from build123d import *

# Parameters (mm, degrees)
SKETCH3_R           = 3.174999999999997
BOSS_EXTRUDE2_DEPTH = 30
SKETCH3_6_R         = 6.249999999999999
SKETCH3_6_R_2       = 3.174999999999996
BOSS_EXTRUDE3_DEPTH = 15
FILLET1_R           = 10
CHAMFER1_SIZE       = 1


with BuildPart() as part:
    # Sketch3 → Boss-Extrude2 (new body)
    with BuildSketch(Plane(origin=(0, 0, 0), x_dir=(1, 0, 0), z_dir=(0, 1, 0))):
        with BuildLine():
            ThreePointArc((-9.29e-15, 31), (-4.229978997044333, 32.64893733094583), (-6.227967505338837, 36.72567114093955))
            ThreePointArc((-6.227967505338856, 36.72567114093959), (-28.456583505173906, 24.03716612275798), (-37.249999999999986, -3.82e-15))
            Line((-37.25, 0), (-41.75, -5.5e-16))
            Line((-41.75, -5.5e-16), (-41.75, -3.000000000000001))
            Line((-41.75, -3.000000000000001), (-40.25, -3.000000000000001))
            Line((-40.25, -3.000000000000001), (-40.25, -1.5000000000000004))
            Line((-40.25, -1.5000000000000004), (-37.21978640454563, -1.5000000000000004))
            ThreePointArc((-37.21978640454562, -1.5000000000000002), (-36.52259085251633, -7.325493663889764), (-34.919347931756114, -12.969257496902395))
            ThreePointArc((-34.91934793175618, -12.969257496902411), (-37.67210506462307, -21.75000000000005), (-28.691380426417297, -23.75641364403726))
            ThreePointArc((-28.691380426417272, -23.756413644037238), (-16.975861979154317, -33.15693909372066), (-2.5, -37.166012699777184))
            Line((-2.4999999999999982, -37.1660126997772), (-2.4999999999999982, -44.1660126997772))
            Line((-2.4999999999999982, -44.1660126997772), (-3.9999999999999982, -44.1660126997772))
            Line((-3.9999999999999982, -44.1660126997772), (-3.9999999999999982, -45.6660126997772))
            Line((-3.9999999999999982, -45.6660126997772), (1.8e-15, -45.6660126997772))
            Line((1.8e-15, -45.6660126997772), (8.2e-16, -30.99999999999999))
            ThreePointArc((8.2e-16, -30.999999999999986), (-30.999999999999986, -3.39e-15), (-1.128e-14, 30.999999999999993))
        make_face()
        with Locations(Location((-32.25944629097033, -18.62500000000002, 0), (0, 0, 270))):
            Circle(SKETCH3_R, mode=Mode.SUBTRACT)
    extrude(amount=BOSS_EXTRUDE2_DEPTH)

    # Sketch3<6> → Boss-Extrude3 (add)
    with BuildSketch(Plane(origin=(0, 0, 0), x_dir=(1, 0, 0), z_dir=(0, 1, 0))):
        with Locations((-8.14e-15, 37.25)):
            Circle(SKETCH3_6_R)
        with Locations(Location((-8.14e-15, 37.25, 0), (0, 0, 270))):
            Circle(SKETCH3_6_R_2, mode=Mode.SUBTRACT)
    extrude(amount=BOSS_EXTRUDE3_DEPTH)

    # Fillet1
    # the kernel refuses this fillet: 10 mm, written as the material it adds along each edge
    with BuildSketch(Plane(origin=(-28.691380426417282, 0, 23.75641364403725), x_dir=(-0.9506898736636257, 0, 0.3101431348803961), z_dir=(0, 1, 0))) as fillet1_piece_1:
        with BuildLine():
            CenterArc((6.482344939436471, 9.575990594652419), FILLET1_R, 209.4937649075162, 43.761742692679945)
            ThreePointArc((-2.221747837989829, 4.652702169021102), (-1.030276989978153, 2.3648375481367587), (0, 0))
            ThreePointArc((0, 0), (1.8006513720656931, 0.26500587834223527), (3.6013027441313774, -6e-17))
        make_face()
    extrude(amount=30)
    with BuildSketch(Plane(origin=(-34.91934793175615, 0, 12.969257496902403), x_dir=(-0.7439367704475782, 0, 0.6682500142731217), z_dir=(0, 1, 0))) as fillet1_piece_2:
        with BuildLine():
            CenterArc((6.482344939436458, -9.575990594652419), FILLET1_R, 106.74449239980393, 43.76174269267989)
            ThreePointArc((-2.2217478379898448, -4.652702169021106), (-1.0302769899781694, -2.364837548136756), (0, 0))
            ThreePointArc((0, 0), (1.8006513720656803, -0.26500587834223843), (3.601302744131356, 6e-17))
        make_face()
    extrude(amount=30)
    with BuildSketch(Plane(origin=(-6.227967505338847, 0, -36.725671140939575), x_dir=(-0.9719890656078827, 0, 0.23502607586971094), z_dir=(0, 1, 0))) as fillet1_piece_3:
        with BuildLine():
            CenterArc((5.848021683595468, -9.976022963631705), FILLET1_R, 93.96846171792617, 43.7617426926798)
            ThreePointArc((-1.5518361342237537, -3.2497978502371354), (-0.5367780683599742, -1.7390925175521244), (0, 0))
            ThreePointArc((0, 0), (2.5779740557861452, -0.08931446047189494), (5.1559481115722905, 1e-17))
        make_face()
    extrude(amount=15)
    with BuildSketch(Plane(origin=(-37.24999999999999, 0, 1.78e-15), x_dir=(-1, 0, -7.737e-14), z_dir=(0, 1, 0))) as fillet1_piece_4:
        with BuildLine():
            CenterArc((9.164670658683216, -8.845385669716253), FILLET1_R, 117.80520941997419, 51.405137085838774)
            ThreePointArc((-0.6585400627312272, -6.973346374538821), (-0.16500045393500687, -3.5021862698004864), (0, 0))
            Line((0, 0), (4.500000000000192, 0))
        make_face()
    extrude(amount=30)

    # Chamfer1
    chamfer1_edges = [part.edges().sort_by_distance(p)[0] for p in [
        (-7.903771868670522, 0, -37.32519260636591),
        (-38.375294648334496, 0, -2.898249101229199),
        (-38.375294648334496, 30, -2.898249101229199),
        (-36.27645093259372, 0, 11.817729079196308),
        (-36.27645093259372, 30, 11.817729079196308),
        (-30.999999999999986, 0, 5.16e-15),
        (1.31e-15, 0, 38.33300634988859),
        (-2.4999999999999982, 0, 40.6660126997772),
        (-14.640454765554196, 0, 34.25229312407797),
        (-14.640454765554196, 30, 34.25229312407797),
        (-2.4999999999999982, 30, 40.6660126997772),
        (1.31e-15, 30, 38.33300634988859),
        (-30.999999999999986, 30, 5.16e-15),
        (-4.2299789970443324, 30, -32.64893733094583),
        (5.376209478406283, 0, -40.43729848685283),
        (-37.672105064623324, 0, 21.749999999999595),
        (-37.672105064623324, 30, 21.749999999999595),
        (-27.849428165120642, 0, -24.7380648167108),
        (-26.07059740166155, 30, -26.60613559163521),
        (-36.941998560282954, 0, 4.780297310006034),
        (-36.941998560282954, 30, 4.780297310006034),
        (-28.372679063924544, 0, 25.507463527167676),
        (-28.372679063924544, 30, 25.507463527167676),
    ]]
    chamfer(chamfer1_edges, length=CHAMFER1_SIZE)


solid = part.part
Build history of the part. All positions in model axes, mm. A direction names the side the tool comes from. Coordinates: 2 decimals unless noted, no trailing zeros. Order: outer loops, then holes, each group sorted by start corner. A loop starts at its lowest first (then second) coordinate and runs counter-clockwise, first axis right, second up. Notation, with made-up numbers: (76.5, -22) - (112.5, -22) arc R25 cw to (112.5, 17) - close; hole circle Ø1 at (27.25, 44). An arc over 180 degrees is marked (long way). Write each question's results on one line, items separated by ' | '. Start each with the question number.
Item 1: Flat gauge pins, fed straight in: pin 1 (2 mm diameter, centred on x = -18, y = 6, fed in from +Z); pin 2 (2 mm diameter, centred on x = -37.5, y = 13, fed in from +Z); pin 3 (1.7 mm diameter, centred on y = 8, z = 2.5, fed in from +X). Where does each tip first touch, or does it go through?
Item 2: Band-saw the part on A-A on y = 10.5. State how many separate pieces and enclosed holes the cut face has, and give its area (3 significant figures).
Item 3: Wall check: probe 1 along Z at (x, y) = (-3, 27); probe 2 along Z at (x, y) = (-2, 5.5); probe 3 along Z at (x, y) = (-37.5, 26). Give the ranges that are in metal, low to high. Write a range as [from, to].
Item 4: Tool access for faces 4 (the face through (-36.95, 14.8, 4.73)), 5 (the face through (-2.5, 15, 41)), 6 (the face through (0, 15, 38)): list every direction of +Z, -Z, +X, -X, +Y, -Y with a clear straight run to the whole face (end or side of a thin tool).
Item 5: Band-saw the part on B-B on y = 17. Write the cut outline in (x, z) (3 decimals).
Item 6: Mould opens along Z. For faces 1 (the face through (-5.1, 29.27, -33.19)), 2 (the face through (-39, 15, 1.5)), 3 (the face through (-3, 15, -39)) say: released by +Z, released by -Z, zero draft, split by the parting line, or undercut.
Numbers:
1) pin 1: z = 33.14 | pin 2: z = 23.22 | pin 3: x = -30.82
2) separate pieces: 1 | enclosed holes: 2 | area: 816 mm^2
3) probe 1: [-31.77, -30.85], [30.85, 37.13], [44.17, 45.67] | probe 2: [-43.17, -39.72], [-34.78, -30.94], [30.94, 45.67] | probe 3: [-4.31, 1.5], [15.21, 22.03]
4) face 4: +Y, -Y | face 5: -X, +Y, -Y | face 6: +Z, +X, +Y, -Y
5) outline: (-41.75, 0) arc R10 cw to (-36.591, -6.973) arc R37.25 ccw to (-6.228, -36.726) arc R6.25 cw to (0, -31) arc R31 cw to (0, 31) - (0, 45.666) - (-4, 45.666) - (-4, 44.166) - (-2.5, 44.166) - (-2.5, 37.166) arc R37.25 ccw to (-25.136, 27.491) arc R10 cw to (-32.115, 24.873) arc R6.25 ccw to (-37.598, 15.376) arc R10 cw to (-36.376, 8.023) arc R37.25 ccw to (-37.22, 1.5) - (-40.25, 1.5) - (-40.25, 3) - (-41.75, 3) - close; hole circle Ø6.35 at (-32.259, 18.625)
6) face 1: released by -Z | face 2: undercut | face 3: zero draft
